CAD build for the part. Positions are in the model's coordinates, mm. A direction names the side the tool comes from. Round coordinates to 2 decimals unless told otherwise and drop trailing zeros. Write each loop counter-clockwise with the first axis right and the second up, starting at its lowest first coordinate (ties: lowest second). Pieces come first, ordered by that corner, then holes. Notation, with made-up numbers: (81.25, 35.25) - (126.25, 35.25) arc R23 cw to (126.25, 73.25) - close; hole circle Ø9 at (52.25, -28.75). An arc over 180 degrees is marked (long way). Put each result on its own line as item: value. Start each with the question number.
Item 1: Cut at B-B (z = 17). Give the cut face in (x, y).
Item 2: Cut at A-A (y = 0). Give the cut face in (x, z), and give its area (3 significant figures).
Item 3: Cut at D-D (z = 27.5). Give the cut face in (x, y).
Item 4: Pin check, flat tips, straight feed: pin 1 Ø5.5 at (x, z) = (28.5, 9) entering from +Y; pin 2 Ø4 at (x, y) = (41, -1) entering from +Z; pin 3 Ø17.5 at (x, z) = (38.5, 5.5) entering from -Y. Stop position of each tip, or through.
Item 5: Drill centre lines: line 1 (Y direction, x = 31.5, z = 0); line 2 (Z direction, x = 34.25, y = 8.5); line 3 (X direction, y = -29.5, z = 28.5). Where is each one in solid material? Low to high. Write a range as from..to.
Item 6: Mould opens along Z. For faces 5 (the flat face through (39, 0, -1.413)), 6 (the cylindrical face through (53.54, 0.31, 20.89)), 7 (the flat face through (54, 32.296, 22)), 8 (the flat face through (54, 0, 29.52)) say: released by +Z, released by -Z, zero draft, split by the parting line, or undercut.
Item 7: 3-axis set-ups, long thin cutter, end or side, ignore diameter. For faces 1 (the flat face through (31, -2, 9)), 2 (the cylindrical face through (53.46, -27.73, 3.52)), 3 (the cylindrical face through (48.6, -0.72, 11.74)), 4 (the flat face through (39, 9.1, 7)): which of +Z, -Z, +X, -X, +Y, -Y reach the whole face in a straight line?
Item 8: Cut at C-C (x = 36.5). Give the cut face in (y, z), and give its area (3 significant figures).
```python
from build123d import *

# Parameters (mm, degrees)
SKETCH_W        = 64.59174
SKETCH_H        = 30.810671
SKETCH_R        = 2.389077
SKETCH_R_2      = 2.369482
PAD001_DEPTH    = 5
SKETCH001_W     = 18.2
SKETCH001_H     = 16
PAD002_DEPTH    = 25
SKETCH002_W     = 14.5
SKETCH002_H     = 12.3
POCKET_DEPTH    = 5
SKETCH003_R     = 3.1
POCKET001_DEPTH = 25.001
SKETCH004_R     = 5.5
POCKET002_DEPTH = 15
FILLET_R        = 16


with BuildPart() as part:
    # Sketch → Pad001 (new body)
    with BuildSketch(Plane(origin=(0, 0, 0), x_dir=(0, -1, 0), z_dir=(-1, 0, 0))):
        with Locations((0, 14.114935)):
            Rectangle(SKETCH_W, SKETCH_H)
        with Locations((-25.982353, 22.020271)):
            Circle(SKETCH_R, mode=Mode.SUBTRACT)
        with Locations((26.01334, 22.020271)):
            Circle(SKETCH_R_2, mode=Mode.SUBTRACT)
        with Locations((0, 18.520271)):
            Circle(SKETCH_R, mode=Mode.SUBTRACT)
    extrude(amount=PAD001_DEPTH)

    # Sketch001 (on Face9 of Pad001) → Pad002 (join)
    with BuildSketch(Plane(origin=(-5, 0, -1.2), x_dir=(0, 1, 0), z_dir=(-1, 0, 0))):
        with Locations((0, -7.786735)):
            Rectangle(SKETCH001_W, SKETCH001_H)
    extrude(amount=PAD002_DEPTH)

    # Sketch002 (on Face15 of Pad002) → Pocket (cut)
    with BuildSketch(Plane(origin=(-30, 0, 0), x_dir=(0, 1, 0), z_dir=(-1, 0, 0))):
        with Locations((0, -6.436735)):
            Rectangle(SKETCH002_W, SKETCH002_H)
    extrude(amount=-POCKET_DEPTH, mode=Mode.SUBTRACT)

    # Sketch003 (on Face20 of Pocket) → Pocket001 (cut, through all)
    with BuildSketch(Plane(origin=(-25, 0, 0), x_dir=(0, 1, 0), z_dir=(-1, 0, 0))):
        with Locations((0, -6.286735)):
            Circle(SKETCH003_R)
    extrude(amount=-POCKET001_DEPTH, mode=Mode.SUBTRACT)

    # Sketch004 (on Face4 of Pocket001) → Pocket002 (cut)
    with BuildSketch(Plane.YZ):
        with Locations((0, 6.286735)):
            Circle(SKETCH004_R)
    extrude(amount=-POCKET002_DEPTH, mode=Mode.SUBTRACT)

    # Fillet
    fillet_edges = [part.edges().sort_by_distance(p)[0] for p in [
        (-2.5, -32.29587, -1.2904),
        (-2.5, 32.29587, -1.2904),
    ]]
    fillet(fillet_edges, radius=FILLET_R)


with BuildPart() as part_1:
    # Body placement: moved
    add(part.part.moved(Location((56, 0, 0))))


solid = part_1.part
```
Output values:
1. outline: (51, -32.3) - (56, -32.3) - (56, -1.84) - (51, -1.84) - close; (51, 1.84) - (56, 1.84) - (56, 32.3) - (51, 32.3) - close
2. outline: (26, -1.41) - (51, -1.41) - (51, -1.29) - (56, -1.29) - (56, 0.79) - (41, 0.79) - (41, 3.19) - (31, 3.19) - (31, 0.29) - (26, 0.29) - close; (26, 12.59) - (31, 12.59) - (31, 9.39) - (41, 9.39) - (41, 11.79) - (56, 11.79) - (56, 16.13) - (51, 16.13) - (51, 14.59) - (26, 14.59) - close; (51, 20.91) - (56, 20.91) - (56, 29.52) - (51, 29.52) - close
2. area: 242 mm2
3. outline: (51, -32.3) - (56, -32.3) - (56, 32.3) - (51, 32.3) - close
4. pin 1: y = 9.1
4. pin 2: z = 14.59
4. pin 3: y = -9.1
5. line 1: -9.1..9.1
5. line 2: -1.41..14.59
5. line 3: 51..56
6. face 5: released by -Z
6. face 6: undercut
6. face 7: zero draft
6. face 8: released by +Z
7. face 1: -X
7. face 2: -Z, +X, -X, -Y
7. face 3: +X
7. face 4: +Z, -Z, -X, +Y
8. outline: (-9.1, -1.41) - (9.1, -1.41) - (9.1, 14.59) - (-9.1, 14.59) - close; hole circle Ø6.2 at (0, 6.29)
8. area: 261 mm2
